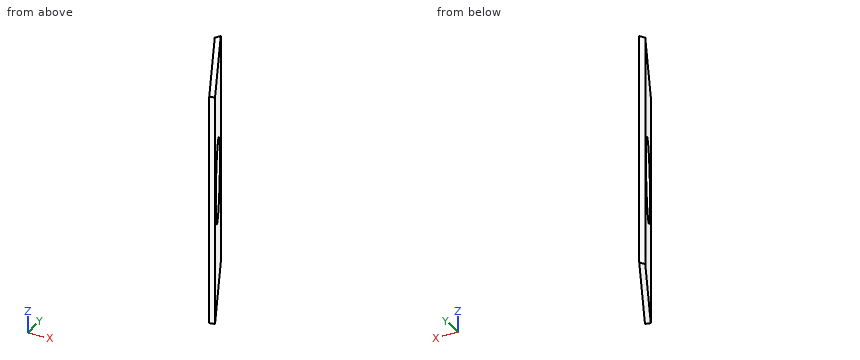
from build123d import *

# Parameters (mm, degrees)
AUFSATZ_LINEAR_AUSTRAGEN1_DEPTH  = 450
F_15_0_15_DURCHMESSER_BOHRUNG1_D = 150


with BuildPart() as part:
    # Skizze1 → Aufsatz-Linear austragen1 (new body)
    with BuildSketch(Plane.XY):
        Polygon((253.156995608, 264.02367356), (246.858259494, 254.02367356), (331.858259494, 76.52367356), (341.858259494, 78.794563683), align=None)
    extrude(amount=AUFSATZ_LINEAR_AUSTRAGEN1_DEPTH)

    # Ø15.0 (15) Durchmesser Bohrung1 (through all)
    with Locations(Plane(origin=(299.762083925, 143.548040189, 0), x_dir=(0, 0, 1), z_dir=(-0.901919134, -0.431904938, 0))):
        with Locations((225, 24.086944564)):
            Hole(F_15_0_15_DURCHMESSER_BOHRUNG1_D / 2)


solid = part.part
Verification items for the finished model (mm, model axes). Coordinates: 2 decimals unless noted, no trailing zeros. Order: outer loops, then holes, each group sorted by start corner. A loop starts at its lowest first (then second) coordinate and runs counter-clockwise, first axis right, second up. Notation, with made-up numbers: M 49,-13.75 L 69,-13.75 A24 cw 69,14.25 Z; hole C -31,72 d11. An arc over 180 degrees is marked long. One line per item, written item: value. Start each with the question number.
Item 1: Sectioned sample at B-B (z = 230). Enter the section's corners in (x, y), then the cut area to 3 significant figures.
Item 2: Sectioned sample at A-A (z = 283.5). Enter the section's corners in (x, y), then the cut area to 3 significant figures.
Item 3: Scan lines: probe 1 along X at (y, z) = (95.5, 322); probe 2 along Y at (x, z) = (275.5, 166.5); probe 3 along X at (y, z) = (107.5, 321). Record each from-to range of solid material in increasing order.
Item 4: Sectioned sample at C-C (z = 374). Enter the section's corners in (x, y).
Item 5: Gauge pin test, flat ends, axial feed: pin 1 (1.5 mm diameter, centred on y = 207.5, z = 336.5, fed in from +X); pin 2 (5 mm diameter, centred on x = 292, z = 137, fed in from -Y); pin 3 (1 mm diameter, centred on y = 236.5, z = 333.5, fed in from +X). Record the tip position at first contact, or that the pin passes through.
Conclusion:
1. outline: M 246.86,254.02 L 257.04,232.77 L 266.06,237.09 L 253.16,264.02 Z; M 321.68,97.78 L 331.86,76.52 L 341.86,78.79 L 330.7,102.1 Z
1. area: 514 mm^2
2. outline: M 246.86,254.02 L 269.09,207.6 L 278.11,211.92 L 253.16,264.02 Z; M 309.63,122.94 L 331.86,76.52 L 341.86,78.79 L 318.65,127.26 Z
2. area: 1,070 mm^2
3. probe 1: x = 322.77 to 333.86
3. probe 2: y = 210.67 to 217.37
3. probe 3: x = 317.02 to 328.11
4. outline: M 246.86,254.02 L 331.86,76.52 L 341.86,78.79 L 253.16,264.02 Z
5. pin 1: stops at x = 280.58
5. pin 2: stops at y = 154.54
5. pin 3: stops at x = 266.58
